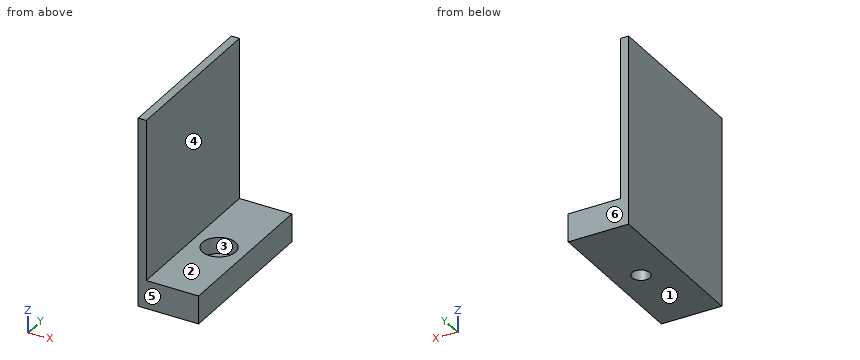
```python
from build123d import *

# Parameters (mm, degrees)
F0_W           = 15
F0_H           = 40
F1_DEPTH       = 7
F2_W           = 2
F2_H           = 40
F3_DEPTH       = 40
F5_D           = 4.4
F5_CBORE_D     = 8.25
F5_CBORE_DEPTH = 4


with BuildPart() as f1:
    # F0 (on Top) → F1 (new body)
    with BuildSketch(Plane.XY):
        Rectangle(F0_W, F0_H)
    extrude(amount=F1_DEPTH)

    # F2 (on face) → F3 (join)
    with BuildSketch(Plane.XY.offset(7)):
        with Locations((-6.5, 0)):
            Rectangle(F2_W, F2_H)
    extrude(amount=F3_DEPTH)

    # F5 (through all)
    with Locations(Plane.XY.offset(7)):
        with Locations((1, 0)):
            CounterBoreHole(F5_D / 2, F5_CBORE_D / 2, F5_CBORE_DEPTH)


solid = f1.part
```
The model under review builds one solid part; all positions refer to its coordinate system, in mm. Face numbers are marked on the shaded views. A direction names the side the tool comes from. Round coordinates to 2 decimals unless told otherwise and drop trailing zeros. Order: outer loops, then holes, each group sorted by start corner. A loop starts at its lowest first (then second) coordinate and runs counter-clockwise, first axis right, second up.
Item 1: Machinability: for the marked faces 1 and 2, which of the approach directions +Z, -Z, +X, -X, +Y, -Y give a long, thin tool a straight path to every point of the face, cutting with its end or side? Answer none if there is none.
Working result:
face 1: -Z, +X, -X, +Y, -Y
face 2: +Z, +X, +Y, -Y
Item 2: For pin 1 (9 mm diameter, centred on x = 0, y = 0.5, fed in from +Z); pin 2 (5.5 mm diameter, centred on x = 1, y = 0, fed in from +Z); pin 3 (3 mm diameter, centred on y = -14.5, z = 15.5, fed in from +X), all flat-tipped, find the tip position at first contact; note any pin that passes through.
Working result:
pin 1: stops at z = 7
pin 2: stops at z = 3
pin 3: stops at x = -5.5
Item 3: Add section B-B, the plane y = 0. State the section outline as (x, z) points (3 decimals).
Working result:
outline: (-7.5, 0) - (-1.2, 0) - (-1.2, 3) - (-3.125, 3) - (-3.125, 7) - (-5.5, 7) - (-5.5, 47) - (-7.5, 47) - close; (3.2, 0) - (7.5, 0) - (7.5, 7) - (5.125, 7) - (5.125, 3) - (3.2, 3) - close
Item 4: To check wall thickness, follow probe 1 along Y at (x, z) = (1, 3.9) (3 decimals); probe 2 along Y at (x, z) = (1, 1.95); probe 3 along Z at (x, y) = (-0.25, -13.5). State the ranges of each line that lie inside material, in increasing order.
Working result:
probe 1: y = -20 to -4.125, 4.125 to 20
probe 2: y = -20 to -2.2, 2.2 to 20
probe 3: z = 0 to 7
Item 5: Add section C-C, the plane y = 9. State the section outline as (x, z) points, and give its area (3 significant figures).
Working result:
outline: (-7.5, 0) - (7.5, 0) - (7.5, 7) - (-5.5, 7) - (-5.5, 47) - (-7.5, 47) - close
area: 185 mm2
Item 6: Add section D-D, the plane z = 14. State the section outline as (x, y) points, and give its area (3 significant figures).
Working result:
outline: (-7.5, -20) - (-5.5, -20) - (-5.5, 20) - (-7.5, 20) - close
area: 80.0 mm2
Item 7: Draft analysis for pull direction Y (two halves, no side actions). For the marked faces 3, 4, 5 and 6, state which applies: released by +Y, released by -Y, zero draft, split by the parting line, or undercut.
Working result:
face 3: undercut
face 4: zero draft
face 5: released by -Y
face 6: released by +Y
Item 8: Add section A-A, the plane x = 1. State the section outline as (y, z) points (3 decimals), and give its area (3 significant figures).
Working result:
outline: (-20, 0) - (-2.2, 0) - (-2.2, 3) - (-4.125, 3) - (-4.125, 7) - (-20, 7) - close; (2.2, 0) - (20, 0) - (20, 7) - (4.125, 7) - (4.125, 3) - (2.2, 3) - close
area: 234 mm2
